Build history of the part. All positions in model axes, mm. A direction names the side the tool comes from. Coordinates: 2 decimals unless noted, no trailing zeros. Write each loop counter-clockwise with the first axis right and the second up, starting at its lowest first coordinate (ties: lowest second). Pieces come first, ordered by that corner, then holes.
```python
from build123d import *

# Parameters (mm, degrees)
F1_DEPTH    = 17.018
F3_DEPTH    = 17.272
F4_W        = 11.0760657117
F4_H        = 15.8854108304
F4_W_2      = 11.9504909962
F5_DEPTH    = 19.812
F6_T4_DEPTH = 141.7175615003


# Not quite as in the source:
# - a fillet or chamfer that OpenCascade refuses, or shapes differently, is made with other operations: its cross-section is extruded or revolved along the edge and cut away or added
# - a feature of the source that left no trace in its solid (it failed there, or was rolled back) is left out


with BuildPart() as f1:
    # F0 (on Front) → F1 (new body)
    with BuildSketch(Plane.XZ):
        Polygon((-58.5865564644, 22.0063943416), (-58.5865564644, -16.7598351836), (38.4747292797, -16.7598351836), (38.4747292797, 22.0063943416), (29.1475392878, 38.0375422537), (-49.2593459785, 38.0375422537), align=None)
    extrude(amount=F1_DEPTH)

    # F2 (on Top) → F3 (join)
    with BuildSketch(Plane.XY):
        Polygon((-58.5865564644, 14.7195085883), (-58.5865564644, 0), (38.4747572243, 0), (38.4747572243, 14.7195085883), (-2.6232791133, 40.3693430126), align=None)
    extrude(amount=-F3_DEPTH)

    # F4 (on face) → F5 (join)
    with BuildSketch(Plane(origin=(0, 0, 0), x_dir=(-1, 0, 0), z_dir=(0, 1, 0))):
        with Locations((-14.282295946, 7.9427054152)):
            Rectangle(F4_W, F4_H)
        with Locations((33.6654121056, 7.9427054152)):
            Rectangle(F4_W_2, F4_H)
    extrude(amount=F5_DEPTH)

    # F6: chamfer of 25.4 on 1 edges, made by hand


with BuildPart() as f6_tool2:
    # F6_s3 → F6_t4 (new body)
    with BuildSketch(Plane.YZ.offset(-56.5764848041)):
        Polygon((19.812, -9.5145891696), (-5.588, 15.8854108304), (19.812, 15.8854108304), align=None)
    extrude(amount=F6_T4_DEPTH)

    split(bisect_by=Plane.XY, keep=Keep.TOP)

    split(bisect_by=Plane.XZ, keep=Keep.BOTTOM)


with BuildPart() as f1_1:
    add(f1.part)

    # F6_t1: cut F6_tool2
    add(f6_tool2.part, mode=Mode.SUBTRACT)


solid = f1_1.part
```
1. Saw through at B-B on x = 14.5. List the corners of the cut face in (y, z).
Computed values:
outline: (-17.02, -16.76) - (0, -16.76) - (0, -17.27) - (29.68, -17.27) - (29.68, 0) - (10.3, 0) - (0, 10.3) - (0, 38.04) - (-17.02, 38.04) - close
2. Probe line 1 along Y through (x, z) = (-33, 12); line 2 along Z through (x, y) = (7, 16.5); line 3 along Z through (x, y) = (-14, -4.5). List the from-to ranges inside material, lowest first.
Computed values:
line 1: y = -17.02 to 0
line 2: z = -17.27 to 0
line 3: z = -16.76 to 38.04
3. 3-axis set-ups, long thin cutter, end or side, ignore diameter. For faces 1 (the face through (-39.641, 4, 4)), 2 (the face through (-11, 0, 19)), 3 (the face through (19.82, 4, 4)), 4 (the face through (-10, 0, -17)), 5 (the face through (-58.587, -4, -2)): which of +Z, -Z, +X, -X, +Y, -Y reach the whole face in a straight line?
Computed values:
face 1: +Z, -X, +Y
face 2: +Z, +Y
face 3: +Z, +X, +Y
face 4: -Z, +X, -X, -Y
face 5: +Z, -Z, -X, +Y, -Y
4. Mould opens along X. For faces 6 (the face through (-53.86, -8.39, 30.13)), 7 (the face through (14.2, 5.2, 5.1)), 8 (the face through (8.744, 4, 4)), 9 (the face through (38.475, -8, 2)) say: +X half, -X half, draft (parallel to the pull), parting line (faces both ways), or undercut.
Computed values:
face 6: -X half
face 7: draft
face 8: undercut
face 9: +X half
5. Flat gauge pins, fed straight in: pin 1 (11.5 mm diameter, centred on x = 4, z = 24, fed in from +Y); pin 2 (18.5 mm diameter, centred on x = -25.5, y = -10.5, fed in from -Z); pin 3 (1 mm diameter, centred on y = 17, z = -1.5, fed in from -X). Where does each tip first touch, or does it go through?
Computed values:
pin 1: stops at y = 0
pin 2: stops at z = -16.76
pin 3: stops at x = -54.7
6. Saw through at D-D on z = 6. List the corners of the cut face in (x, y), plus the area to 3 significant figures.
Computed values:
outline: (-58.59, -17.02) - (38.47, -17.02) - (38.47, 0) - (19.82, 0) - (19.82, 4.3) - (8.74, 4.3) - (8.74, 0) - (-27.69, 0) - (-27.69, 4.3) - (-39.64, 4.3) - (-39.64, 0) - (-58.59, 0) - close
area: 1,750 mm2
7. Saw through at C-C on y = -6. List the corners of the cut face in (x, z).
Computed values:
outline: (-58.59, -16.76) - (38.47, -16.76) - (38.47, 22.01) - (29.15, 38.04) - (-49.26, 38.04) - (-58.59, 22.01) - close
